from build123d import *

# Parameters (mm, degrees)
CROQUIS1_R              = 1.55
SALIENTE_EXTRUIR1_DEPTH = 7
REDONDEO1_R             = 1
REDONDEO2_R             = 2
CROQUIS2_R              = 1.55
CORTAR_EXTRUIR1_DEPTH   = 33.110590153
CROQUIS3_W              = 8
CROQUIS3_H              = 7
CROQUIS3_R              = 1.55
SALIENTE_EXTRUIR2_DEPTH = 5


with BuildPart() as part:
    # Croquis1 → Saliente-Extruir1 (new body)
    # profile 1 of 3: a face of its own
    with BuildSketch(Plane.XY):
        with BuildLine():
            ThreePointArc((-9.7, 5), (-14.7, 0), (-9.7, -5))
            Line((-9.7, -5), (-29.7, -5))
            Line((-29.7, -5), (-29.7, 5))
            Line((-29.7, 5), (-9.7, 5))
        make_face()
    # profile 2 of 3: a face of its own
    with BuildSketch(Plane.XY):
        with BuildLine():
            Line((14.282575695, 2), (-9.7, 2))
            Line((-9.7, 2), (-14.282575695, 2))
            ThreePointArc((-14.282575695, 2), (-13.883300133, -2.738612788), (-9.7, -5))
            Line((-9.7, -5), (9.7, -5))
            ThreePointArc((9.7, -5), (13.883300133, -2.738612788), (14.282575695, 2))
        make_face()
        with Locations((-9.7, 0)):
            Circle(CROQUIS1_R, mode=Mode.SUBTRACT)
        with Locations((9.7, 0)):
            Circle(CROQUIS1_R, mode=Mode.SUBTRACT)
    # profile 3 of 3: a face of its own
    with BuildSketch(Plane.XY):
        with BuildLine():
            Line((-9.7, 2), (-9.7, 5))
            ThreePointArc((-9.7, 5), (-12.438612788, 4.183300133), (-14.282575695, 2))
            Line((-14.282575695, 2), (-9.7, 2))
        make_face()
    extrude(amount=SALIENTE_EXTRUIR1_DEPTH)

    # Redondeo1
    redondeo1_edges = [part.edges().sort_by_distance(p)[0] for p in [
        (14.282575695, 2, 3.5),
    ]]
    fillet(redondeo1_edges, radius=REDONDEO1_R)

    # Redondeo2
    redondeo2_edges = [part.edges().sort_by_distance(p)[0] for p in [
        (-9.7, 5, 3.5),
    ]]
    fillet(redondeo2_edges, radius=REDONDEO2_R)

    # Croquis2 → Cortar-Extruir1 (cut, through all)
    with BuildSketch(Plane(origin=(0, 5, 0), x_dir=(1, 0, 0), z_dir=(0, 1, 0))):
        with Locations(Location((-25.7, -3.5, 0), (0, 0, 180))):
            Circle(CROQUIS2_R)
    extrude(amount=-CORTAR_EXTRUIR1_DEPTH, mode=Mode.SUBTRACT)

    # Croquis3 → Saliente-Extruir2 (add)
    with BuildSketch(Plane.XZ.offset(5)):
        with Locations((-25.7, 3.5)):
            Rectangle(CROQUIS3_W, CROQUIS3_H)
        with Locations(Location((-25.7, 3.5, 0), (0, 0, 180))):
            Circle(CROQUIS3_R, mode=Mode.SUBTRACT)
    extrude(amount=SALIENTE_EXTRUIR2_DEPTH)


solid = part.part
Build history of the part. All positions in model axes, mm. A direction names the side the tool comes from. Coordinates: 2 decimals unless noted, no trailing zeros. Write each loop counter-clockwise with the first axis right and the second up, starting at its lowest first coordinate (ties: lowest second). Pieces come first, ordered by that corner, then holes.
(1) Cut at D-D on y = -6.5. List the corners of the cut face in (x, z).
(2) 3-axis set-ups, long thin cutter, end or side, ignore diameter. For faces 5 (the flat face through (-13, -1, 7)), 6 (the flat face through (-9.7, 2.5, 3.5)), 7 (the flat face through (-6, -5, 3)): which of +Z, -Z, +X, -X, +Y, -Y reach the whole face in a straight line?
(3) Cut at B-B on y = 0. List the corners of the cut face in (x, z), and give its area (3 significant figures).
(4) Cut at A-A on z = 3.5. List the corners of the cut face in (x, y).
(5) Pin check, flat tips, straight feed: pin 1 Ø1.5 at (y, z) = (-1, 4.5) entering from +X; pin 2 Ø4 at (x, y) = (9.7, 0) entering from +Z; pin 3 Ø2 at (x, z) = (-10, 5) entering from -Y; pin 4 Ø4 at (y, z) = (-7.5, 2.5) entering from +X. Stop position of each tip, or through.
(6) Mould opens along X. For faces 1 (the cylindrical face through (-8.222, 0.466, 3.451)), 2 (the flat face through (2, 2, 3)), 3 (the cylindrical face through (11.178, 0.466, 3.451)), 4 (the flat face through (-29.7, -2, 3)) say: pulls with the +X half, pulls with the -X half, needs draft (parallel to the pull), parting line crosses it, or undercut.
(7) Cut at C-C on x = -25.7. List the corners of the cut face in (y, z).
(8) Drill centre lines: line 1 (Z direction, x = -25.7, y = -4.25); line 2 (Y direction, x = 9.7, z = 2.75); line 3 (Y direction, x = -4, z = 2.25). Where is each one in solid material? Low to high.
Working result:
1. outline: (-29.7, 0) - (-21.7, 0) - (-21.7, 7) - (-29.7, 7) - close; hole circle Ø3.1 at (-25.7, 3.5)
2. face 5: +Z, +X, -X, +Y, -Y
2. face 6: +Z, -Z, +X, +Y
2. face 7: +Z, -Z, +X, -Y
3. outline: (-29.7, 0) - (-11.25, 0) - (-11.25, 7) - (-29.7, 7) - close; (-8.15, 0) - (8.15, 0) - (8.15, 7) - (-8.15, 7) - close; (11.25, 0) - (14.7, 0) - (14.7, 7) - (11.25, 7) - close; hole circle Ø3.1 at (-25.7, 3.5)
3. area: 260 mm2
4. outline: (-29.7, -10) - (-27.25, -10) - (-27.25, 5) - (-29.7, 5) - close; (-24.15, -10) - (-21.7, -10) - (-21.7, -5) - (9.7, -5) arc R5 ccw to (14.54, 1.25) arc R1 ccw to (13.57, 2) - (-9.7, 2) - (-9.7, 3) arc R2 ccw to (-11.7, 5) - (-24.15, 5) - close; hole circle Ø3.1 at (-9.7, 0); hole circle Ø3.1 at (9.7, 0)
5. pin 1: stops at x = 14.69
5. pin 2: stops at z = 7
5. pin 3: stops at y = -5
5. pin 4: stops at x = -21.7
6. face 1: undercut
6. face 2: needs draft
6. face 3: undercut
6. face 4: pulls with the -X half
7. outline: (-10, 0) - (5, 0) - (5, 1.95) - (-10, 1.95) - close; (-10, 5.05) - (5, 5.05) - (5, 7) - (-10, 7) - close
8. line 1: z = 0 to 1.95, 5.05 to 7
8. line 2: y = -5 to -1.55, 1.55 to 2
8. line 3: y = -5 to 2
